Check sheet for the modelled part. Datum: model origin and axes. Units: mm. A direction names the side the tool comes from. Round coordinates to 2 decimals unless told otherwise and drop trailing zeros. Write each loop counter-clockwise with the first axis right and the second up, starting at its lowest first coordinate (ties: lowest second). Pieces come first, ordered by that corner, then holes. Notation, with made-up numbers: (61.25, -40) -> (92.25, -40) arc R12 ccw to (92.25, -20) -> close; hole circle Ø5 at (-10, -9.5). An arc over 180 degrees is marked (long way). Use one line per item in the form item = value. Start each with the question number.
Autodesk Inventor part; units mm, degrees
ref_plane "YZ Plane" through (0, 0, 0) normal (1, 0, 0) x (0, 1, 0)
ref_plane "XZ Plane" through (0, 0, 0) normal (0, 1, 0) x (-1, 0, 0)
ref_plane "XY Plane" through (0, 0, 0) normal (0, 0, 1) x (1, 0, 0)
sketch "Sketch1" plane through (0, 0, 0) normal (0, 1, 0) x (-1, 0, 0)
  line L0 (0, 0) -> (50.8, 0)
  line L1 (50.8, 0) -> (50.8, -25.4)
  line L2 (50.8, -25.4) -> (0, -25.4)
  line L3 (0, -25.4) -> (0, 0)
  line L4 (48.26, -22.86) -> (48.26, -2.54)
  line L5 (48.26, -2.54) -> (2.54, -2.54)
  line L6 (2.54, -2.54) -> (2.54, -22.86)
  line L7 (2.54, -22.86) -> (48.26, -22.86)
  dimension "d0" = 50.8
  dimension "d1" = 25.4
  dimension "d2" = 2.54
extrude "Extrusion1" add sketch "Sketch1" along normal blind 11.43
extrude "Extrusion2" add sketch "Sketch1" along normal blind 1.27 contours L7 L6 L5 L4
sketch "Sketch2" plane through (0, 11.43, 0) normal (0, 1, 0) x (1, 0, 0)
  line L0 (-48.26, 22.86) -> (-2.54, 22.86)
  line L1 (-2.54, 22.86) -> (-2.54, 2.54)
  line L2 (-2.54, 2.54) -> (-48.26, 2.54)
  line L3 (-48.26, 2.54) -> (-48.26, 22.86)
  line L4 (-50.8, 0) -> (0, 0)
  line L5 (0, 0) -> (0, 25.4)
  line L6 (0, 25.4) -> (-50.8, 25.4)
  line L7 (-50.8, 25.4) -> (-50.8, 0)
  line L8 (-49.53, 24.13) -> (-1.27, 24.13)
  line L9 (-1.27, 24.13) -> (-1.27, 1.27)
  line L10 (-1.27, 1.27) -> (-49.53, 1.27)
  line L11 (-49.53, 1.27) -> (-49.53, 24.13)
  dimension "d7" = 1.27
extrude "Extrusion3" cut sketch "Sketch2" against normal blind 1.27 contours L8 L9 L10 L11
fillet "Fillet1" radius 1.27 12 edges at (-2.54, 5.715, -2.54) (-1.27, 10.795, -1.27) (0, 5.715, 0) (-50.8, 5.715, 0) (-49.53, 10.795, -1.27) (-48.26, 5.715, -2.54) (-50.8, 5.715, -25.4) (-49.53, 10.795, -24.13) (-48.26, 5.715, -22.86) (0, 5.715, -25.4) (-1.27, 10.795, -24.13) (-2.54, 5.715, -22.86)
sketch "Sketch3" plane through (0, 0, 0) normal (0, -1, 0) x (1, 0, 0)
  circle A0 centre (-53.975, 3.175) radius 1.8415
  circle A1 centre (-12.065, 3.175) radius 1.8415
  circle A2 centre (-53.975, 3.175) radius 3.81
  circle A3 centre (-12.065, 3.175) radius 3.81
  line L0 (-1.27, 0) -> (-49.53, 0)
  line L1 (-56.6691, 0.4809) -> (-50.8, -5.3882)
  line L2 (-51.2809, 5.8691) -> (-45.4118, 0)
  line L3 (-15.8678, 2.941) -> (-15.8678, 0)
  line L4 (-8.255, 3.175) -> (-8.255, 0)
  arc A4 (-1.27, -25.4) -> (0, -24.13) centre (-1.27, -24.13) ccw
  line L5 (0, -24.13) -> (0, -1.27)
  arc A5 (0, -1.27) -> (-1.27, 0) centre (-1.27, -1.27) ccw
  line L6 (-1.27, 0) -> (-49.53, 0)
  arc A6 (-49.53, 0) -> (-50.8, -1.27) centre (-49.53, -1.27) ccw
  line L7 (-50.8, -1.27) -> (-50.8, -24.13)
  arc A7 (-50.8, -24.13) -> (-49.53, -25.4) centre (-49.53, -24.13) ccw
  line L8 (-49.53, -25.4) -> (-1.27, -25.4)
  line L9 (-50.8, -24.13) -> (-50.8, -1.27)
  line L10 (-50.8, -5.3882) -> (-50.8, -1.27)
  arc A8 (-49.53, 0) -> (-50.8, -1.27) centre (-49.53, -1.27) ccw
  line L11 (-49.53, 0) -> (-45.4118, 0)
  point P0 (0, 0)
  dimension "d11" = 3.683
  dimension "d13" = 41.91
  dimension "d14" = 7.62
  dimension "d16" = 3.175
  dimension "d17" = 45
extrude "Extrusion4" add sketch "Sketch3" against normal blind 2.54 contours A2 | A2 L2 L0 A6 L7 L1 | L3 A3 L0 | A3 L0 | A3 L4 L0 picked at (-11.991, 0.449)
fillet "Fillet2" radius 1.905 4 edges at (-8.255, 1.27, 0) (-15.8678, 1.27, 0) (-45.4118, 1.27, 0) (-50.8, 1.27, -5.3882)
properties part number "BackupNanoCasePart1" material "ABS Plastic"
1. Sectioned sample at D-D (x = -54). Enter the section's corners in (y, z), and give its area (3 significant figures).
2. Sectioned sample at B-B (x = -28.5). Enter the section's corners in (y, z).
3. Sectioned sample at A-A (y = 6.5). Enter the section's corners in (x, z).
4. Scan lines: probe 1 along X at (y, z) = (6, -17); probe 2 along Z at (x, y) = (-23.5, 10); probe 3 along Z at (x, y) = (-37, 10.75). Record each from-to range of solid material in increasing order.
5. Depth check by flat-ended pin: pin 1 (3.5 mm diameter, centred on x = -10, z = 2.5, fed in from +Y); pin 2 (2 mm diameter, centred on x = -19, z = -14, fed in from +Y); pin 3 (3 mm diameter, centred on x = -53.975, z = 3.175, fed in from +Y); pin 4 (1.4 mm diameter, centred on y = 10.5, z = -13, fed in from -X). Enter the tip coordinate at first touch or a pass-through.
6. Sectioned sample at C-C (z = -13). Enter the section's corners in (x, y), and give its area (3 significant figures).
7. Mould release check, pull along X, two halves, no side actions. Record for faces 1 (the face through (-50.95, 1.29, -5.44)), 2 (the face through (-7.68, 1.29, 0.54)), 3 (the face through (-28, 0, -13)), 4 (the face through (-49.148, 10.786, -1.632)): +X half, -X half, draft (parallel to the pull), parting line (faces both ways), or undercut.
8. Tool access check on faces 5 (the face through (-50.8, 6, -13)), 6 (the face through (-21.9, 10.16, -23.8)), 7 (the face through (-12, 2.54, 1)). Record the directions out of +Z, -Z, +X, -X, +Y, -Y that give a thin tool (end or side, any length) a straight path to the whole face; none if there is none.
Returned:
q1.outline = (0, -2.19) -> (2.54, -2.19) -> (2.54, 1.33) -> (0, 1.33) -> close; (0, 5.02) -> (2.54, 5.02) -> (2.54, 6.98) -> (0, 6.98) -> close
q1.area = 13.9 mm^2
q2.outline = (0, -25.4) -> (11.43, -25.4) -> (11.43, -24.13) -> (10.16, -24.13) -> (10.16, -22.86) -> (1.27, -22.86) -> (1.27, -2.54) -> (10.16, -2.54) -> (10.16, -1.27) -> (11.43, -1.27) -> (11.43, 0) -> (0, 0) -> close
q3.outline = (-50.8, -24.13) arc R1.27 ccw to (-49.53, -25.4) -> (-1.27, -25.4) arc R1.27 ccw to (0, -24.13) -> (0, -1.27) arc R1.27 ccw to (-1.27, 0) -> (-49.53, 0) arc R1.27 ccw to (-50.8, -1.27) -> close; hole (-48.26, -21.59) arc R1.27 ccw to (-46.99, -22.86) -> (-3.81, -22.86) arc R1.27 ccw to (-2.54, -21.59) -> (-2.54, -3.81) arc R1.27 ccw to (-3.81, -2.54) -> (-46.99, -2.54) arc R1.27 ccw to (-48.26, -3.81) -> close
q4.probe_1 = -50.8 to -48.26, -2.54 to 0
q4.probe_2 = -25.4 to -22.86, -2.54 to 0
q4.probe_3 = -25.4 to -24.13, -1.27 to 0
q5.pin_1 = 2.54
q5.pin_2 = 1.27
q5.pin_3 = through
q5.pin_4 = -50.8
q6.outline = (-50.8, 0) -> (0, 0) -> (0, 11.43) -> (-1.27, 11.43) -> (-1.27, 10.16) -> (-2.54, 10.16) -> (-2.54, 1.27) -> (-48.26, 1.27) -> (-48.26, 10.16) -> (-49.53, 10.16) -> (-49.53, 11.43) -> (-50.8, 11.43) -> close
q6.area = 113 mm^2
q7.face_1 = -X half
q7.face_2 = +X half
q7.face_3 = draft
q7.face_4 = undercut
q8.face_5 = -Z, -X, +Y
q8.face_6 = +Y
q8.face_7 = +Z, +X, -X, +Y
